```python
from build123d import *

# Parameters (mm, degrees)
SKETCH1_R               = 3
BOSS_EXTRUDE1_DEPTH     = 12.5
CUT_EXTRUDE4_DEPTH      = 9
CUT_EXTRUDE4_DEPTH_BACK = 9


with BuildPart() as part:
    # Sketch1 → Boss-Extrude1 (new body)
    with BuildSketch(Plane(origin=(0, 0, 0), x_dir=(1, 0, 0), z_dir=(0, 1, 0))):
        Circle(SKETCH1_R)
    extrude(amount=BOSS_EXTRUDE1_DEPTH)

    # Sketch3 → Revolve1 (revolve)
    with BuildSketch(Plane.XY):
        Polygon((-3, 12.5), (-8, 17.5), (0, 17.5), (0, 12.5), align=None)
    revolve(axis=Axis((0, 17.5, 0), (0, -1, 0)))

    # Sketch4 → Cut-Extrude4 (cut, two sides)
    with BuildSketch(Plane.XY) as cut_extrude4_sk:
        Polygon((0.588175988, 67.243680335), (0.588175988, 17.501049711), (0.588175988, 16.5), (-1.411824012, 16.5), (-1.411824012, 17.501049711), (-1.411824012, 67.243680335), (-1.411824012, 166.728941583), (0.588175988, 166.728941583), align=None)
    extrude(amount=CUT_EXTRUDE4_DEPTH, mode=Mode.SUBTRACT)
    extrude(cut_extrude4_sk.sketch, amount=-CUT_EXTRUDE4_DEPTH_BACK, mode=Mode.SUBTRACT)

    # Sketch6 → Revolve2 (revolve)
    with BuildSketch(Plane.XY):
        Polygon((3, 0), (0, -1.732050808), (0, 0), align=None)
    revolve(axis=Axis((0, -1.732050808, 0), (0, 1, 0)))


solid = part.part
```
The listing builds one solid part. Answer for the finished solid, in the listing's coordinates (mm). A direction names the side the tool comes from. Coordinates: 2 decimals unless noted, no trailing zeros. Write each loop counter-clockwise with the first axis right and the second up, starting at its lowest first coordinate (ties: lowest second). Pieces come first, ordered by that corner, then holes. Notation, with made-up numbers: M 58.5,43.25 L 79.5,43.25 A26 cw 79.5,74.25 Z; hole C -20.75,85 d8. An arc over 180 degrees is marked long. Use a Markdown table: item, result. Add a question column.
1. For a pull along X with two mould halves and no side action, classify faces 1 (the flat face through (-4, 17.5, 0)), 2 (the flat face through (0.588, 17, 0)), 3 (the conical face through (-0.38, -1.456, 0.291)) as +X half, -X half, draft (parallel to the pull), parting line (faces both ways), or undercut.
2. Given P1, Ø0.5, axis at y = 17, z = -1.5, coming from the -X side; P2, Ø4, axis at x = 6.5, z = -5.5, coming from the -Y side; P3, Ø4, axis at y = 14.5, z = -1, coming from the -X side, each flat-ended and moving along its own axis, determine where each tip first touches the part or whether it passes through.
3. Straight lines are drawn through the part: line 1 along X through (y, z) = (12.25, 0); line 2 along Y through (x, z) = (-2.5, -5.25); line 3 along Y through (x, z) = (1.25, 2.5). For each, find the intervals that lie inside material, in ascending order. Write a range as [from, to].
4. Which of the six approach directions +Z, -Z, +X, -X, +Y, -Y give full straight-line access (tool end or side, diameter ignored) to faces 4 (the flat face through (0, 16.5, 0)), 5 (the cylindrical face through (-3, 6, 0)), 6 (the flat face through (4, 17.5, 0))?
5. Section A-A (y = 8) is taken. Give the vertices of the cut face in (x, z), plus the area to 3 significant figures.
Data:
| question | item | result |
|---|---|---|
| 1 | face 1 | draft |
| 1 | face 2 | undercut |
| 1 | face 3 | parting line |
| 2 | P1 | stops at x = -7.61 |
| 2 | P2 | stops at y = 16.01 |
| 2 | P3 | stops at x = -6.94 |
| 3 | line 1 | x = [-3, 3] |
| 3 | line 2 | y = [15.31, 17.5] |
| 3 | line 3 | y = [-0.12, 17.5] |
| 4 | face 4 | +Z, -Z, +Y |
| 4 | face 5 | -Y |
| 4 | face 6 | +Z, -Z, +X, -X, +Y |
| 5 | outline | C 0,0 d6 |
| 5 | area | 28.3 mm2 |
